from build123d import *

# Parameters (mm, degrees)
SKETCH1_W               = 74.5
SKETCH1_H               = 75
BOSS_EXTRUDE1_DEPTH     = 55
SKETCH5_R               = 34.3615522135402
CUT_EXTRUDE2_DEPTH      = 100.90745717913153
BOSS_EXTRUDE3_DEPTH     = 74.5
BOSS_EXTRUDE4_DEPTH     = 74.5
CUT_EXTRUDE3_DEPTH      = 121.88656873284145
CUT_EXTRUDE3_DEPTH_BACK = 121.88656873284145
SKETCH9_W               = 64.5
SKETCH9_H               = 49.00000000000001
BOSS_EXTRUDE5_DEPTH     = 3
BOSS_EXTRUDE6_DEPTH     = 3
FILLET1_R               = 1
SKETCH12_R              = 2.499999999999999
SKETCH12_R_2            = 2.5000000000000027
SKETCH12_R_3            = 2.5000000000000018
CUT_EXTRUDE4_DEPTH      = 91.13219475054404
LPATTERN1_COUNT         = 2
LPATTERN1_PITCH         = 104.2


with BuildPart() as part:
    # Sketch1 → Boss-Extrude1 (new body)
    with BuildSketch(Plane(origin=(0, 0, 0), x_dir=(1, 0, 0), z_dir=(0, 1, 0))):
        Rectangle(SKETCH1_W, SKETCH1_H)
    extrude(amount=BOSS_EXTRUDE1_DEPTH)

    # Sketch5 → Cut-Extrude2 (cut, through all)
    with BuildSketch(Plane(origin=(37.25, 0, 0), x_dir=(0, 0, -1), z_dir=(1, 0, 0))):
        with Locations((6.94e-15, 55)):
            Circle(SKETCH5_R)
    extrude(amount=-CUT_EXTRUDE2_DEPTH, mode=Mode.SUBTRACT)

    # Sketch7 → Boss-Extrude3 (add)
    with BuildSketch(Plane(origin=(37.25, 0, 0), x_dir=(0, 0, -1), z_dir=(1, 0, 0))):
        Polygon((-37.49999999999999, 55), (-63.5, 0), (-37.49999999999999, 0), align=None)
    extrude(amount=-BOSS_EXTRUDE3_DEPTH)

    # Sketch8 → Boss-Extrude4 (add)
    with BuildSketch(Plane(origin=(37.25, 0, 0), x_dir=(0, 0, -1), z_dir=(1, 0, 0))):
        Polygon((37.50000000000001, 55), (63.5, -2.4e-16), (37.50000000000001, 0), align=None)
    extrude(amount=-BOSS_EXTRUDE4_DEPTH)

    # Sketch9 → Cut-Extrude3 (cut, two sides: drawn at the far end of the back side and taken through both)
    with BuildSketch(Plane.XY.offset(37.49999999999999).offset(-CUT_EXTRUDE3_DEPTH_BACK)):
        with Locations((0, 27.500000000000004)):
            Rectangle(SKETCH9_W, SKETCH9_H)
    extrude(amount=CUT_EXTRUDE3_DEPTH + CUT_EXTRUDE3_DEPTH_BACK, mode=Mode.SUBTRACT)

    # Sketch10 → Boss-Extrude5 (add)
    with BuildSketch(Plane(origin=(0, 55, 0), x_dir=(1, 0, 0), z_dir=(0, 1, 0))):
        with BuildLine():
            ThreePointArc((6.164042343036378, 37.499999999999844), (7.158223158465123, 39.534270662732936), (7.5, 41.77253812074898))
            ThreePointArc((7.5, 41.77253812074898), (-2.2382674580157964, 48.93076127921418), (-6.164042343036669, 37.50000000000026))
            Line((-6.164042343036755, 37.50000000000001), (-2.5971942566442934, 37.50000000000001))
            ThreePointArc((-2.5971942566443156, 37.499999999999936), (-2.4509211244732474, 46.1306323879271), (4.999999999999999, 41.77253812074898))
            ThreePointArc((4.999999999999999, 41.77253812074898), (4.358094267178168, 39.32161699627582), (2.5971942566444843, 37.50000000000004))
            Line((2.5971942566444923, 37.50000000000001), (6.164042343036321, 37.50000000000001))
        make_face()
    extrude(amount=-BOSS_EXTRUDE5_DEPTH)

    # Sketch11 → Boss-Extrude6 (add)
    with BuildSketch(Plane(origin=(0, 55, 0), x_dir=(1, 0, 0), z_dir=(0, 1, 0))):
        with BuildLine():
            ThreePointArc((-6.023640204727232, -37.49999999999989), (-2.3529448000904902, -49.08965777094965), (7.5, -41.96830601951038))
            ThreePointArc((7.5, -41.96830601951038), (7.121351751439286, -39.615361219419945), (6.023640204727302, -37.499999999999986))
            Line((6.0236402047273, -37.49999999999999), (2.2437115046296583, -37.49999999999999))
            ThreePointArc((2.243711504629653, -37.500000000000014), (4.255499825117389, -39.34328768844565), (4.999999999999999, -41.96830601951038))
            ThreePointArc((4.999999999999999, -41.96830601951038), (-2.6250183310647546, -46.223805844627755), (-2.2437115046296032, -37.49999999999999))
            Line((-2.2437115046296014, -37.49999999999999), (-6.023640204727201, -37.49999999999999))
        make_face()
        with BuildLine():
            Line((2.2437115046296583, -37.49999999999999), (6.0236402047273, -37.49999999999999))
            ThreePointArc((6.023640204727302, -37.499999999999986), (5.875e-14, -34.46830601951038), (-6.023640204727232, -37.49999999999989))
            Line((-6.023640204727201, -37.49999999999999), (-2.2437115046296014, -37.49999999999999))
            ThreePointArc((-2.2437115046296032, -37.49999999999999), (2.806e-14, -36.96830601951038), (2.243711504629653, -37.500000000000014))
        make_face()
    extrude(amount=-BOSS_EXTRUDE6_DEPTH)

    # Fillet1
    # the kernel refuses this fillet: 1 mm, written as the material it takes off along each edge
    with BuildSketch(Plane(origin=(-3.55e-15, 55, 41.96830601951038), x_dir=(1, 0, 0), z_dir=(0, 0, -1))) as fillet1_piece_1_section:
        with BuildLine():
            CenterArc((7.5 - FILLET1_R, FILLET1_R), FILLET1_R, 270, 90)
            Line((7.5, FILLET1_R), (7.5, 0))
            Line((7.5, 0), (7.5 - FILLET1_R, 0))
        make_face()
    fillet1_piece_1 = revolve(axis=Axis((-3.55e-15, 55, 41.96830601951038), (0, -1, 0)), revolution_arc=235.71091499042655, mode=Mode.PRIVATE)
    fillet1_piece_1 = split(fillet1_piece_1, bisect_by=Plane(origin=(-2.6713999236626833, 50.45322927533666, 39.6493825243863), z_dir=(0, 0.42737961689341636, 0.9040722665053036)), keep=Keep.TOP, mode=Mode.PRIVATE)
    add(fillet1_piece_1, mode=Mode.SUBTRACT)
    with BuildSketch(Plane(origin=(1.78e-15, 52, 41.96830601951038), x_dir=(-0.7297482724094352, 0, -0.6837159197469698), z_dir=(0.6837159197469698, 0, -0.7297482724094352))) as fillet1_piece_2_section:
        with BuildLine():
            CenterArc((7.500000000000202 - FILLET1_R, FILLET1_R), FILLET1_R, 270, 90)
            Line((7.500000000000198, FILLET1_R), (7.500000000000202, 0))
            Line((7.500000000000202, 0), (7.500000000000202 - FILLET1_R, 0))
        make_face()
    fillet1_piece_2 = revolve(axis=Axis((1.78e-15, 52, 41.96830601951038), (0, 1, 0)), revolution_arc=223.13470500677207, mode=Mode.PRIVATE)
    fillet1_piece_2 = split(fillet1_piece_2, bisect_by=Plane(origin=(-1.7477354157855842, 48.3431338081412, 40.64688219978779), z_dir=(0, 0.42737961689341636, 0.9040722665053036)), keep=Keep.TOP, mode=Mode.PRIVATE)
    add(fillet1_piece_2, mode=Mode.SUBTRACT)
    with BuildSketch(Plane(origin=(1.33e-15, 55, -41.772538120748976), x_dir=(-0.5894081060524027, 0, 0.8078354315822744), z_dir=(0.8078354315822744, 0, 0.5894081060524027))) as fillet1_piece_3_section:
        with BuildLine():
            CenterArc((7.500000000001482 - FILLET1_R, FILLET1_R), FILLET1_R, 270, 90)
            Line((7.500000000001481, FILLET1_R), (7.500000000001482, 0))
            Line((7.500000000001482, 0), (7.500000000001482 - FILLET1_R, 0))
        make_face()
    fillet1_piece_3 = revolve(axis=Axis((1.33e-15, 55, -41.772538120748976), (0, -1, 0)), revolution_arc=287.7699662913145, mode=Mode.PRIVATE)
    fillet1_piece_3 = split(fillet1_piece_3, bisect_by=Plane(origin=(0, 50.33119352274253, -39.70707215288535), z_dir=(0, 0.42737961689341614, -0.9040722665053037)), keep=Keep.TOP, mode=Mode.PRIVATE)
    add(fillet1_piece_3, mode=Mode.SUBTRACT)
    with BuildSketch(Plane(origin=(5.33e-15, 52, -41.77253812074899), x_dir=(0.7487686990913793, 0, 0.662831377697981), z_dir=(-0.662831377697981, 0, 0.7487686990913793))) as fillet1_piece_4_section:
        with BuildLine():
            CenterArc((7.499999999999997 - FILLET1_R, FILLET1_R), FILLET1_R, 269.9999999999997, 90.00000000000028)
            Line((7.499999999999997 - FILLET1_R, 0), (7.499999999999997, 0))
            Line((7.499999999999997, 0), (7.499999999999996, FILLET1_R))
        make_face()
    fillet1_piece_4 = revolve(axis=Axis((5.33e-15, 52, -41.77253812074899), (0, 1, 0)), revolution_arc=263.03233782444397, mode=Mode.PRIVATE)
    fillet1_piece_4 = split(fillet1_piece_4, bisect_by=Plane(origin=(7.11e-15, 48.33525291032238, -40.65060771512034), z_dir=(0, 0.42737961689341614, -0.9040722665053037)), keep=Keep.TOP, mode=Mode.PRIVATE)
    add(fillet1_piece_4, mode=Mode.SUBTRACT)
    with BuildSketch(Plane(origin=(1.78e-15, 52, 41.96830601951038), x_dir=(1, 0, 0), z_dir=(0, 0, 1))) as fillet1_piece_5_section:
        with BuildLine():
            CenterArc((7.499999999999997 - FILLET1_R, FILLET1_R), FILLET1_R, 270, 90)
            Line((7.499999999999998, FILLET1_R), (7.499999999999997, 0))
            Line((7.499999999999997, 0), (7.499999999999997 - FILLET1_R, 0))
        make_face()
    fillet1_piece_5 = revolve(axis=Axis((1.78e-15, 52, 41.96830601951038), (0, 1, 0)), revolution_arc=43.0957883273494, mode=Mode.PRIVATE)
    fillet1_piece_5 = split(fillet1_piece_5, bisect_by=Plane(origin=(7.034955474041542, 51.63351194574045, 39.09143071655905), z_dir=(0, 0.42737961689341636, 0.9040722665053036)), keep=Keep.TOP, mode=Mode.PRIVATE)
    add(fillet1_piece_5, mode=Mode.SUBTRACT)
    with BuildSketch(Plane(origin=(-3.55e-15, 55, 41.96830601951038), x_dir=(0.563991699397745, 0, -0.825780456907551), z_dir=(-0.825780456907551, 0, -0.563991699397745))) as fillet1_piece_6_section:
        with BuildLine():
            CenterArc((7.499999999999998 - FILLET1_R, FILLET1_R), FILLET1_R, 270, 90)
            Line((7.499999999999998, FILLET1_R), (7.499999999999998, 0))
            Line((7.499999999999998, 0), (7.499999999999998 - FILLET1_R, 0))
        make_face()
    fillet1_piece_6 = revolve(axis=Axis((-3.55e-15, 55, 41.96830601951038), (0, -1, 0)), revolution_arc=55.66769762264099, mode=Mode.PRIVATE)
    fillet1_piece_6 = split(fillet1_piece_6, bisect_by=Plane(origin=(6.774695529731854, 53.96765158354673, 37.988019251414265), z_dir=(0, 0.42737961689341636, 0.9040722665053036)), keep=Keep.TOP, mode=Mode.PRIVATE)
    add(fillet1_piece_6, mode=Mode.SUBTRACT)

    # Sketch12 → Cut-Extrude4 (cut, through all)
    with BuildSketch(Plane(origin=(0, 3, 0), x_dir=(1, 0, 0), z_dir=(0, 1, 0))):
        with Locations(Location((-17.25, -52.08181818181816, 0), (0, 0, 270))):
            Circle(SKETCH12_R)
        with Locations(Location((17.25, -52.081818181818164, 0), (0, 0, 270))):
            Circle(SKETCH12_R_2)
        with Locations(Location((0, -52.081818181818164, 0), (0, 0, 270))):
            Circle(SKETCH12_R_3)
    cut_extrude4 = extrude(amount=-CUT_EXTRUDE4_DEPTH, mode=Mode.SUBTRACT)

    # LPattern1: Cut-Extrude4 ×2
    with Locations(*[(0, 0, -i * LPATTERN1_PITCH) for i in range(1, LPATTERN1_COUNT)]):
        add(cut_extrude4, mode=Mode.SUBTRACT)


solid = part.part
Geometry check sheet. Reference: the model listing, model coordinates, mm. A direction names the side the tool comes from. Round coordinates to 2 decimals unless told otherwise and drop trailing zeros. Loops run counter-clockwise (first coordinate to the right, second up) from the corner with the lowest first, then second, coordinate; pieces in that order, holes last. Notation, with made-up numbers: (62, 36.5) - (115, 36.5) arc R25 cw to (115, 61.5) - close; hole circle Ø3 at (75.5, 74.5). An arc over 180 degrees is marked (long way). Answer as CSV lines item,"result".
(1) Cross-section at C-C, the plane x = 30. Enter the section's corners in (y, z).
Output values:
outline,"(0, -63.5) - (3, -62.08) - (3, 62.08) - (0, 63.5) - close; (52, -38.92) - (55, -37.5) - (55, -34.36) arc R34.36 cw to (52, -34.23) - close; (52, 34.23) arc R34.36 cw to (55, 34.36) - (55, 37.5) - (52, 38.92) - close"
(2) Cross-section at B-B, the plane z = -36. Enter the section's corners in (x, y), and give its area (3 significant figures).
Output values:
outline,"(-37.25, 0) - (37.25, 0) - (37.25, 55) - (-37.25, 55) - close; hole (-32.25, 3) - (32.25, 3) - (32.25, 52) - (-32.25, 52) - close"
area,"937 mm²"
(3) Depth check by flat-ended pin: pin 1 Ø6 at (x, z) = (0, -41.77) entering from +Y. Enter the tip coordinate at first touch or a pass-through.
Output values:
pin 1,"stops at y = 52.31"
(4) Set-up check for faces 1 (the face through (0, 52, -37)), 2 (the face through (37.25, 16, -1)), 3 (the face through (0.06, 53.52, 38.2)): record each of +Z, -Z, +X, -X, +Y, -Y from which the full face is reachable in a straight line by a thin tool's end or side.
Output values:
face 1,"+Z, -Z"
face 2,"+Z, -Z, +X, +Y, -Y"
face 3,"+Y"
(5) Cross-section at D-D, the plane y = 6. Enter the section's corners in (x, z).
Output values:
outline,"(-37.25, -60.66) - (-32.25, -60.66) - (-32.25, 60.66) - (-37.25, 60.66) - close; (32.25, -60.66) - (37.25, -60.66) - (37.25, 60.66) - (32.25, 60.66) - close"
(6) Release check for a two-part mould opening along Z. For faces 4 (the face through (0, 52, 38)), 5 (the face through (-0.96, 1.52, 54.39)) record: released by +Z, released by -Z, zero draft, split by the parting line, or undercut.
Output values:
face 4,"zero draft"
face 5,"undercut"
(7) Material ranges on line 1 along X through (y, z) = (22, -48); line 2 along Y through (x, z) = (3, -7), recorded low to high.
Output values:
line 1,"x = -37.25 to -32.25, 32.25 to 37.25"
line 2,"y = 0 to 3"
(8) Cross-section at A-A, the plane x = 0. Give the number of separate pieces and of enclosed holes in the cut face, and give its area (3 significant figures).
Output values:
separate pieces,"7"
enclosed holes,"0"
area,"384 mm²"
